from build123d import *

# Parameters (mm, degrees)
SKETCH1_R           = 6.5
BOSS_EXTRUDE1_DEPTH = 5.8
SKETCH2_R           = 4
CUT_EXTRUDE1_DEPTH  = 93.260613645
FILLET1_R           = 0.5
SKETCH3_R           = 4.775
CUT_EXTRUDE2_DEPTH  = 1.5875


with BuildPart() as part:
    # Sketch1 → Boss-Extrude1 (new body)
    with BuildSketch(Plane.XY):
        with Locations((85.206527413, -1.763997815)):
            Circle(SKETCH1_R)
    extrude(amount=BOSS_EXTRUDE1_DEPTH)

    # Sketch2 → Cut-Extrude1 (cut, through all)
    with BuildSketch(Plane.XY.offset(5.8)):
        with Locations((85.206527413, -1.763997815)):
            Circle(SKETCH2_R)
    extrude(amount=-CUT_EXTRUDE1_DEPTH, mode=Mode.SUBTRACT)

    # Fillet1
    fillet1_edges = [part.edges().sort_by_distance(p)[0] for p in [
        (81.206527413, -1.763997815, 5.8),
    ]]
    fillet(fillet1_edges, radius=FILLET1_R)

    # Sketch3 → Cut-Extrude2 (cut)
    with BuildSketch(Plane(origin=(0, 0, 0), x_dir=(-1, 0, 0), z_dir=(0, 0, -1))):
        with Locations((-85.206527413, -1.763997815)):
            Circle(SKETCH3_R)
    extrude(amount=-CUT_EXTRUDE2_DEPTH, mode=Mode.SUBTRACT)


solid = part.part
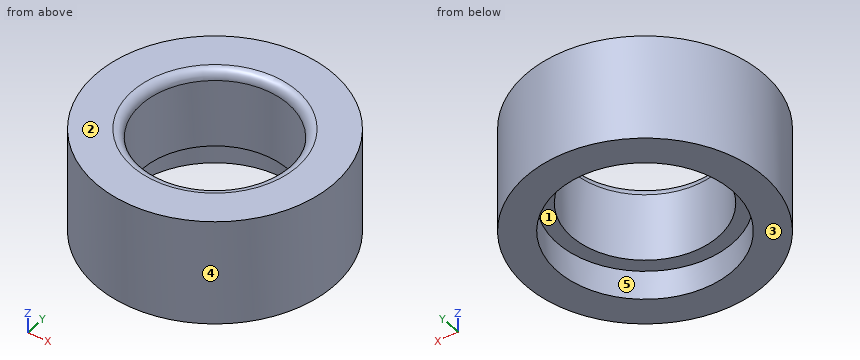
Read the model definition and answer for the solid it produces. Units are mm, in the model's axes. Face numbers are marked on the shaded views. A direction names the side the tool comes from. Coordinates: 2 decimals unless noted, no trailing zeros. Loops run counter-clockwise (first coordinate to the right, second up) from the corner with the lowest first, then second, coordinate; pieces in that order, holes last. Notation, with made-up numbers: (-28, -13) -> (25, -13) arc R37 ccw to (25, 24) -> close; hole circle Ø6 at (78, 57). An arc over 180 degrees is marked (long way). Answer in a Markdown table with one row per item.
Item 1: Straight lines are drawn through the part: line 1 along Y through (x, z) = (87.25, 5.2); line 2 along X through (y, z) = (-4, 0.4); line 3 along Y through (x, z) = (82.5, 3). For each, find the intervals that lie inside material, in ascending order. Write a range as [from, to].
Returned:
| item | result |
|---|---|
| line 1 | y = [-7.93, -5.2], [1.67, 4.41] |
| line 2 | x = [79.1, 80.99], [89.43, 91.31] |
| line 3 | y = [-7.67, -4.71], [1.18, 4.15] |
Item 2: For the marked faces 1 and 2, determine the directions among +Z, -Z, +X, -X, +Y, -Y from which every point of the face is accessible in a straight line to the end or side of a thin tool.
Returned:
| item | result |
|---|---|
| face 1 | -Z |
| face 2 | +Z, +X, -X, +Y, -Y |
Item 3: Each of these flat-tipped pins is pushed along its axis until it touches: P1, Ø1, axis at x = 86.5, z = 4.5, coming from the -Y side; P2, Ø1.5, axis at y = -5.5, z = 2, coming from the +X side; P3, Ø6, axis at x = 85, y = -1, coming from the -Z side; P4, Ø1, axis at y = -4, z = 1, coming from the -X side. Where does it stop, or does it pass through?
Returned:
| item | result |
|---|---|
| P1 | stops at y = -8.22 |
| P2 | stops at x = 90.98 |
| P3 | passes through |
| P4 | stops at x = 78.94 |
Item 4: A cutting plane is placed at B-B on y = 4.25. Determine the outline of the cut face in (x, z).
Returned:
| item | result |
|---|---|
| outline | (82.74, 0) -> (87.67, 0) -> (87.67, 5.8) -> (82.74, 5.8) -> close |
Item 5: A cutting plane is placed at D-D on z = 3.2. Determine the outline of the cut face in (x, y), plus the area to 3 significant figures.
Returned:
| item | result |
|---|---|
| outline | circle Ø13 at (85.21, -1.76); hole circle Ø8 at (85.21, -1.76) |
| area | 82.5 mm^2 |
Item 6: For a pull along X with two mould halves and no side action, classify the marked faces 3, 4 and 5 as released by +X, released by -X, zero draft, split by the parting line, or undercut.
Returned:
| item | result |
|---|---|
| face 3 | zero draft |
| face 4 | split by the parting line |
| face 5 | undercut |
Item 7: A cutting plane is placed at C-C on x = 79.5. Determine the outline of the cut face in (y, z).
Returned:
| item | result |
|---|---|
| outline | (-4.88, 0) -> (1.35, 0) -> (1.35, 5.8) -> (-4.88, 5.8) -> close |
Item 8: A cutting plane is placed at A-A on z = 0.5. Determine the outline of the cut face in (x, y) (3 decimals), plus the area to 3 significant figures.
Returned:
| item | result |
|---|---|
| outline | circle Ø13 at (85.207, -1.764); hole circle Ø9.55 at (85.207, -1.764) |
| area | 61.1 mm^2 |
